Verification items for the finished model (mm, model axes). A direction names the side the tool comes from. Coordinates: 2 decimals unless noted, no trailing zeros. Write each loop counter-clockwise with the first axis right and the second up, starting at its lowest first coordinate (ties: lowest second). Pieces come first, ordered by that corner, then holes. Notation, with made-up numbers: (32.5, 44) -> (62.5, 44) arc R21 ccw to (62.5, 48) -> close; hole circle Ø4 at (18, -13). An arc over 180 degrees is marked (long way). Answer in a Markdown table with one row per item.
```python
from build123d import *

# Parameters (mm, degrees)
F1_DEPTH      = 30
F1_DEPTH_BACK = 10
F1_TAPER_BACK = -3


with BuildPart() as f1:
    # F0 (on Front) → F1 (new body, two sides)
    with BuildSketch(Plane.XZ) as f1_sk:
        Polygon((-17.5708103925, 27.9494225979), (-27.0390175283, 0), (-17.3887293786, -36.5072265267), (0, -36.5072265267), (16.2962432951, -36.5072265267), (28.1315054744, 0), (19.2095395178, 27.9494225979), align=None)
    extrude(amount=F1_DEPTH)
    extrude(f1_sk.sketch, amount=-F1_DEPTH_BACK, taper=F1_TAPER_BACK)


solid = f1.part
```
1. Tool access check on faces 1 (the flat face through (-1, -15, -36.507)), 2 (the flat face through (-22.28, -14.79, -18)), 3 (the flat face through (1, -15, 27.949)). Record the directions out of +Z, -Z, +X, -X, +Y, -Y that give a thin tool (end or side, any length) a straight path to the whole face; none if there is none.
Geometry says:
| item | result |
|---|---|
| face 1 | -Z, +X, -X, -Y |
| face 2 | -Z, -X, -Y |
| face 3 | +Z, +X, -X, -Y |
2. Section check A-A, the plane y = -24.5. Record the boundary of the cut face in (x, z), plus the area to 3 significant figures.
Geometry says:
| item | result |
|---|---|
| outline | (-27.04, 0) -> (-17.39, -36.51) -> (16.3, -36.51) -> (28.13, 0) -> (19.21, 27.95) -> (-17.57, 27.95) -> close |
| area | 2,910 mm^2 |
3. Thickness scan on line 1 (Z direction, x = 6, y = -7); line 2 (X direction, y = 0, z = -5); line 3 (Z direction, x = 11.5, y = 5.5). Record the ranges inside material, lowest first. Write a range as from..to.
Geometry says:
| item | result |
|---|---|
| line 1 | -36.51..27.95 |
| line 2 | -25.72..26.51 |
| line 3 | -36.8..28.24 |
4. Depth check by flat-ended pin: P1, Ø2, axis at y = -20, z = 11, coming from the -X side; P2, Ø15, axis at x = 8.5, y = -8, coming from the +Z side; P3, Ø1, axis at y = -20.5, z = -11.5, coming from the +X side. Enter the tip coordinate at first touch or a pass-through.
Geometry says:
| item | result |
|---|---|
| P1 | x = -23.65 |
| P2 | z = 27.95 |
| P3 | x = 24.57 |
